from build123d import *

# Parameters (mm, degrees)
SKETCH1_R           = 1.55
SKETCH1_R_2         = 1.6
BOSS_EXTRUDE1_DEPTH = 3


with BuildPart() as part:
    # Sketch1 → Boss-Extrude1 (new body)
    with BuildSketch(Plane(origin=(0, 0, 0), x_dir=(1, 0, 0), z_dir=(0, 1, 0))):
        Polygon((-40.25, 40), (40.25, 40), (40.25, -40), (40.25, -48), (-48.25, -48), (-48.25, -40), (-48.25, 40), align=None)
        with Locations(Location((-36.2, -35.95, 0), (0, 0, 270))):
            Circle(SKETCH1_R, mode=Mode.SUBTRACT)
        with Locations(Location((-36.2, 22.45, 0), (0, 0, 270))):
            Circle(SKETCH1_R, mode=Mode.SUBTRACT)
        with Locations(Location((20.8, 34.45, 0), (0, 0, 270))):
            Circle(SKETCH1_R, mode=Mode.SUBTRACT)
        with Locations(Location((31.3, -22.45, 0), (0, 0, 270))):
            Circle(SKETCH1_R, mode=Mode.SUBTRACT)
        with Locations(Location((-44.25, 27.75, 0), (0, 0, 270))):
            Circle(SKETCH1_R_2, mode=Mode.SUBTRACT)
        with Locations(Location((-44.25, -27.75, 0), (0, 0, 270))):
            Circle(SKETCH1_R_2, mode=Mode.SUBTRACT)
        with Locations(Location((-35.74, -44, 0), (0, 0, 270))):
            Circle(SKETCH1_R, mode=Mode.SUBTRACT)
        with Locations(Location((-23.74, -44, 0), (0, 0, 270))):
            Circle(SKETCH1_R, mode=Mode.SUBTRACT)
    extrude(amount=BOSS_EXTRUDE1_DEPTH)


solid = part.part
Input: part model. Units: mm. Frame: model coordinates. Give positions to 0.01 mm unless a question says otherwise; leave off trailing zeros. Order: outer loops, then holes, each group sorted by start corner. A loop starts at its lowest first (then second) coordinate and runs counter-clockwise, first axis right, second up. Notation, with made-up numbers: (38, 66) -> (47, 66) arc R10 cw to (47, 82) -> close; hole circle Ø2 at (54, 74). An arc over 180 degrees is marked (long way). Use one line per item in the form item = value.
1) Section A-A, the plane x = 20.8. Return loops of the section in (y, z), and give its area (3 significant figures).
Response values:
outline = (0, -40) -> (3, -40) -> (3, -36) -> (0, -36) -> close; (0, -32.9) -> (3, -32.9) -> (3, 48) -> (0, 48) -> close
area = 255 mm^2
2) Line query: probe 1 along Z at (x, y) = (-36, 0.75); probe 2 along X at (y, z) = (0.6, 22.45); probe 3 along X at (y, z) = (1.65, -22.45). Output: solid intervals per line, ascending.
Response values:
probe_1 = -40 to -23.99, -20.91 to 34.41, 37.49 to 42.47, 45.53 to 48
probe_2 = -48.25 to 29.75, 32.85 to 40.25
probe_3 = -48.25 to -37.75, -34.65 to 40.25
3) Section B-B, the plane z = -22.45. Return loops of the section in (x, y).
Response values:
outline = (-48.25, 0) -> (-37.75, 0) -> (-37.75, 3) -> (-48.25, 3) -> close; (-34.65, 0) -> (40.25, 0) -> (40.25, 3) -> (-34.65, 3) -> close
4) First-contact query: pin 1 Ø5 at (x, z) = (-22, 21) entering from -Y. Flat tip, straight axial feed; report the tip coordinate or a pass-through.
Response values:
pin_1 = 0
5) Mould query, pull axis X, two halves, no side actions, for faces 1 (the flat face through (-48.25, 1, 3)), 2 (the flat face through (-3, 1, 48)), 3 (the cylindrical face through (-22.43, 1.48, 44.83)). Classes: pulls with the +X half, pulls with the -X half, needs draft (parallel to the pull), parting line crosses it, or undercut.
Response values:
face_1 = pulls with the -X half
face_2 = needs draft
face_3 = undercut
